Autodesk Inventor part; units mm, degrees
ref_plane "Start Plane" through (0, 0, 19.05) normal (0, 0, 1) x (1, 0, 0)
ref_plane "End Plane" through (0, 0, 666.75) normal (0, 0, 1) x (1, 0, 0)
ref_plane "Work Plane5" through (-406.4, 19.05, 666.75) normal (0, 0, 1) x (1, 0, 0)
ref_plane "Start Plane" through (0, 0, 19.05) normal (0, 0, 1) x (1, 0, 0)
ref_plane "End Plane" through (0, 0, 666.75) normal (0, 0, 1) x (1, 0, 0)
sketch "Sketch" plane through (0, 0, 0) normal (0, 0, 1) x (1, 0, 0)
  line L0 (-19.05, 19.05) -> (19.05, 19.05)
  line L1 (19.05, 19.05) -> (19.05, -19.05)
  line L2 (19.05, -19.05) -> (-19.05, -19.05)
  line L3 (-19.05, -19.05) -> (-19.05, 19.05)
  line L4 (15.875, 15.875) -> (-15.875, 15.875)
  line L5 (-15.875, 15.875) -> (-15.875, -15.875)
  line L6 (-15.875, -15.875) -> (15.875, -15.875)
  line L7 (15.875, -15.875) -> (15.875, 15.875)
  point P0 (0, 0)
  point P1 (0, 19.05)
  point P2 (-19.05, 0)
  dimension "width" = 38.1
  dimension "d1" = 3.175
extrude "Body" add sketch "Sketch" along normal up to surface (647.7 mm away) from surface at 19.05
sketch "Sketch4" plane through (0, 0, 0) normal (0, 0, 1) x (1, 0, 0)
  line L0 (0, 0) -> (10, 0)
ref_plane "Work Plane4" through (0, 0, 0) normal (0, -1, 0) x (1, 0, 0)
sketch "Sketch5" plane through (0, 0, 0) normal (0, -1, 0) x (1, 0, 0)
  line L0 (-2, 19.05) -> (12, 19.05)
  line L1 (-2, 666.75) -> (12, 666.75)
  dimension "d9" = 647.7
ref_plane "Work Plane5" through (-406.4, 19.05, 666.75) normal (0, 0, 1) x (1, 0, 0)
split "Split1" plane through (-406.4, 19.05, 666.75) removes the side toward (0, 0, 1)
ref_plane "Work Plane6" through (762, 19.05, 19.05) normal (0, 0, -1) x (-1, 0, 0)
split "Split2" plane through (762, 19.05, 19.05) removes the side toward (0, 0, -1)
equation "\"G_OFFSET_START\" = -19.05"
equation "\"G_OFFSET_END\" = -19.05"
equation "\"d4\" = -G_OFFSET_START"
equation "\"d5\" = length + G_OFFSET_END"
equation "\"G_L\" = 723.9"
properties part number "1.5x1.5x.125 Tube" material "Aluminum-6061"
Could you check a few things on this model? Use its own coordinates, in mm. A direction names the side the tool comes from. Round coordinates to 2 decimals unless told otherwise and drop trailing zeros. Write each loop counter-clockwise with the first axis right and the second up, starting at its lowest first coordinate (ties: lowest second). Pieces come first, ordered by that corner, then holes.
(1) Suppose I cut it at A-A on x = 9.5. Write out the boundary of the cut face in (y, z) (3 decimals), and give its area (3 significant figures).
Findings below:
outline: (-19.05, 19.05) - (-15.875, 19.05) - (-15.875, 666.75) - (-19.05, 666.75) - close; (15.875, 19.05) - (19.05, 19.05) - (19.05, 666.75) - (15.875, 666.75) - close
area: 4,110 mm2
(2) Suppose I cut it at B-B on z = 181. Write out the boundary of the cut face in (x, y) (3 decimals), and give its area (3 significant figures).
Findings below:
outline: (-19.05, -19.05) - (19.05, -19.05) - (19.05, 19.05) - (-19.05, 19.05) - close; hole (-15.875, -15.875) - (15.875, -15.875) - (15.875, 15.875) - (-15.875, 15.875) - close
area: 444 mm2
(3) Thinking about a two-plate mould opening in Y: for faces 1 (the face through (-17, 0, 666.75)), 2 (the face through (0, -19.05, 338)), 3 (the face through (-15.875, 0, 338)), which applies, +Y half, -Y half, draft (parallel to the pull), parting line (faces both ways), or undercut?
Findings below:
face 1: draft
face 2: -Y half
face 3: undercut
(4) Which directions (+Z, -Z, +X, -X, +Y, -Y) give clear straight access to the entire face, cutting with the end or side of a thin tool? Please do faces 4 (the face through (0, 19.05, 338)), 5 (the face through (0, 15.875, 338)).
Findings below:
face 4: +Z, -Z, +X, -X, +Y
face 5: +Z, -Z
(5) If I drill on probe 1 along Y at (x, z) = (-7, 333) (3 decimals), over which ranges is the centre line in solid material (lowest first)?
Findings below:
probe 1: y = -19.05 to -15.875, 15.875 to 19.05
